Read the model definition and answer for the solid it produces. Units are mm, in the model's axes. A direction names the side the tool comes from. Round coordinates to 2 decimals unless told otherwise and drop trailing zeros. Order: outer loops, then holes, each group sorted by start corner. A loop starts at its lowest first (then second) coordinate and runs counter-clockwise, first axis right, second up. Notation, with made-up numbers: (59, 75) -> (112, 75) arc R8 cw to (112, 79) -> close; hole circle Ø9 at (14.25, 58). An arc over 180 degrees is marked (long way). Answer as a JSON object with one key per item and string values. Group by question number.
Item 1: The mould has two halves that part along Y. Classify faces 3 (the cylindrical face through (0.22, -9.7, 3.22)), 4 (the cylindrical face through (3.711, -5.713, 3.219)), 5 (the flat face through (-14.5, 0, 3)), 6 (the flat face through (8, 15, 3)): pulls with the +Y half, pulls with the -Y half, needs draft (parallel to the pull), parting line crosses it, or undercut.
Item 2: Section A-A, the plane x = -0.5 is taken. Write down the section's boundary in (y, z).
Item 3: Section D-D, the plane x = 7 is taken. Write down the section's boundary in (y, z) (3 decimals), plus the area to 3 significant figures.
Item 4: Given P1, Ø1.5, axis at x = -4, z = 3, coming from the +Y side; P2, Ø4, axis at x = 13.22, y = -11.25, coming from the -Z side; P3, Ø3, axis at x = -4.5, z = 5, coming from the +Y side; P4, Ø2.5, axis at x = -4.49, y = -4.49, coming from the -Z side, each flat-ended and moving along its own axis, determine where each tip first touches the part or whether it passes through.
Item 5: Section B-B, the plane y = -11.25 is taken. Write down the section's boundary in (x, z).
Item 6: Section C-C, the plane z = 0.75 is taken. Count the separate pieces of the cut face and the enclosed holes in it, plus the area to 3 significant figures.
Item 7: Consider probe 1 along Y at (x, z) = (0, 2.25) (3 decimals); probe 2 along X at (y, z) = (11.25, 5.35); probe 3 along X at (y, z) = (10.75, 5). Determine where each line is inside the solid, lowest interval first. Write a range as from..to.
Item 8: For faces 1 (the cylindrical face through (14.143, 10.405, 3.762)), 2 (the flat face through (13, -7.5, 3)), determine the directions among +Z, -Z, +X, -X, +Y, -Y from which every point of the face is accessible in a straight line to the end or side of a thin tool.
from build123d import *

# Parameters (mm, degrees)
F1_DEPTH       = 6.35
F2_D           = 2.5
F2_CSINK_D     = 4.7
F2_CSINK_ANGLE = 90
F3_D           = 2.9
F4_D           = 2
F6_D           = 2.05
F6_DEPTH       = 8
F6_TIP         = 0.6158821345


# Not quite as in the source:
# - ends of sketch curves that miss each other by under 0.0002 mm in the source are joined
# - a length typed as a fraction of an inch, garbled in the dataset ("3 / 203.2 mm" for 3/8 in), is restored


with BuildPart() as f1:
    # F0 (on Top) → F1 (new body)
    with BuildSketch(Plane.XY):
        with BuildLine():
            ThreePointArc((0, -2.5), (-2.5, 0), (0, 2.5))
            Line((0, 2.5), (0, 6.35))
            Line((0, 6.35), (0, 15))
            ThreePointArc((0, 15), (-9.1485355902, 11.8871483777), (-14.5, 3.8405728739))
            Line((-14.5, 3.8405728739), (-14.5, -3.8405728739))
            ThreePointArc((-14.5, -3.8405728739), (-9.1485355902, -11.8871483777), (0, -15))
            Line((0, -15), (0, -2.5))
        make_face()
        with BuildLine():
            ThreePointArc((0, 2.5), (1.767766953, 1.767766953), (2.5, 0))
            ThreePointArc((2.5, 0), (1.767766953, -1.767766953), (0, -2.5))
            Line((0, -2.5), (0, -15))
            Line((0, -15), (16.39699, -15))
            Line((16.39699, -15), (16.39699, -7.5))
            Line((16.39699, -7.5), (10.0469859317, -7.5))
            Line((10.0469859317, -7.5), (10.0469859317, 7.5))
            Line((10.0469859317, 7.5), (16.3969859317, 7.5))
            Line((16.3969859317, 7.5), (16.39699, 15))
            Line((16.39699, 15), (0, 15))
            Line((0, 15), (0, 6.35))
            Line((0, 6.35), (0, 2.5))
        make_face()
    extrude(amount=F1_DEPTH)

    # F2 (through all)
    with Locations(Plane(origin=(0, 0, 0), x_dir=(1, 0, 0), z_dir=(0, 0, -1))):
        with Locations((13.2219879658, -11.25), (13.2219879658, 11.25)):
            CounterSinkHole(F2_D / 2, F2_CSINK_D / 2, counter_sink_angle=F2_CSINK_ANGLE)

    # F3 (through all)
    with Locations(Plane(origin=(0, 0, 0), x_dir=(1, 0, 0), z_dir=(0, 0, -1))):
        with Locations((-4.4901280605, -4.4901280605), (4.4901280605, -4.4901280605), (4.4901280605, 4.4901280605), (-4.4901280605, 4.4901280605)):
            Hole(F3_D / 2)

    # F4 (through all)
    with Locations(Plane(origin=(0, 0, 0), x_dir=(1, 0, 0), z_dir=(0, 0, -1))):
        with Locations((0, -10.675), (-10.675, 0), (0, 10.675)):
            Hole(F4_D / 2)

    # F6
    with Locations(Plane.YZ.offset(10.0469859317)):
        with Locations((0, 3.175)):
            Hole(F6_D / 2, depth=F6_DEPTH)
            with Locations((0, 0, -(F6_DEPTH + F6_TIP / 2))):  # 118° drill point
                Cone(0, F6_D / 2, F6_TIP, mode=Mode.SUBTRACT)


solid = f1.part
Values found:
{
 "1": {"face 3": "undercut", "face 4": "undercut", "face 5": "needs draft", "face 6": "pulls with the +Y half"},
 "2": {"outline": "(-14.99, 0) -> (-11.54, 0) -> (-11.54, 6.35) -> (-14.99, 6.35) -> close; (-9.81, 0) -> (-2.45, 0) -> (-2.45, 6.35) -> (-9.81, 6.35) -> close; (2.45, 0) -> (9.81, 0) -> (9.81, 6.35) -> (2.45, 6.35) -> close; (11.54, 0) -> (14.99, 0) -> (14.99, 6.35) -> (11.54, 6.35) -> close"},
 "3": {"outline": "(-15, 0) -> (15, 0) -> (15, 6.35) -> (-15, 6.35) -> close; hole circle Ø2.05 at (0, 3.175)", "area": "187 mm2"},
 "4": {"P1": "y = 14.64", "P2": "z = 0.35", "P3": "y = 14.7", "P4": "through"},
 "5": {"outline": "(-9.92, 0) -> (-0.82, 0) -> (-0.82, 6.35) -> (-9.92, 6.35) -> close; (0.82, 0) -> (10.87, 0) -> (11.97, 1.1) -> (11.97, 6.35) -> (0.82, 6.35) -> close; (14.47, 1.1) -> (15.57, 0) -> (16.4, 0) -> (16.4, 6.35) -> (14.47, 6.35) -> close"},
 "6": {"separate pieces": "1", "enclosed holes": "10", "area": "676 mm2"},
 "7": {"probe 1": "-15..-11.675, -9.675..-2.5, 2.5..9.675, 11.675..15", "probe 2": "-9.92..-0.82, 0.82..11.97, 14.47..16.4", "probe 3": "-10.46..-1, 1..12.08, 14.37..16.4"},
 "8": {"face 1": "+Z, -Z", "face 2": "+Z, -Z, +X"}
}
